Geometry: final body of the model. Coordinates: model frame, mm. A direction names the side the tool comes from. Give positions to 0.01 mm unless a question says otherwise; leave off trailing zeros. Write each loop counter-clockwise with the first axis right and the second up, starting at its lowest first coordinate (ties: lowest second). Pieces come first, ordered by that corner, then holes. Notation, with made-up numbers: M 12.25,66 L 22.25,66 A30 ccw 22.25,104 Z; hole C -22,65 d5. An arc over 180 degrees is marked long. Use a Markdown table: item, result. Add a question column.
(1) Cut plane D-D (x = 8). Output: boundary loops of the cut face in (y, z), plus the area to 3 significant figures.
(2) Material intervals for L1, parallel to Z at x = 9, y = 19.75; L2, parallel to Z at x = 18, y = 22.75; L3, parallel to X at y = 23.25, z = -15.5, sorted ascending.
(3) Draft query along Y for faces 6 (the flat face through (41.5, 2.5, -2)), 7 (the flat face through (22, 25, -14)), 8 (the flat face through (22, 23, -14)). Return one class per face: released by +Y, released by -Y, zero draft, split by the parting line, or undercut.
(4) Cut plane C-C (y = 14.75). Output: boundary loops of the cut face in (x, z), plus the area to 3 significant figures.
(5) Cut plane A-A (z = -11.5). Output: boundary loops of the cut face in (x, y).
(6) Reachability of faces 1 (the flat face through (44, 3, -14)), 2 (the flat face through (22.7, 22.5, -25)), 3 (the flat face through (41, 24, -26)), 4 (the flat face through (1, 7.21, -14)), 5 (the flat face through (22, 12, 0)) from +Z, -Z, +X, -X, +Y, -Y: full face, straight path, thin tool, end or side. Return the list, or none.
(7) Pin query (flat end, axial travel): pin 1 Ø4 at (y, z) = (18, -23.5) entering from +X; pin 2 Ø0.9 at (x, z) = (41.5, -10.5) entering from +Y. Return the tip coordinate at first contact, or that it passes through.
(8) Cut plane B-B (z = -23). Output: boundary loops of the cut face in (x, y), plus the area to 3 significant figures.
```python
from build123d import *

# Parameters (mm, degrees)
SKETCH1_W           = 45
SKETCH1_H           = 28
BOSS_EXTRUDE1_DEPTH = 3
BOSS_EXTRUDE2_DEPTH = 22
SKETCH4_W           = 45
SKETCH4_H           = 28
SKETCH4_W_2         = 3
SKETCH4_H_2         = 24
BOSS_EXTRUDE4_DEPTH = 2
SKETCH5_W           = 8.5
SKETCH5_H           = 3.5
CUT_EXTRUDE1_DEPTH  = 2
BOSS_EXTRUDE6_DEPTH = 1
SKETCH8_W           = 3
SKETCH8_H           = 24
CUT_EXTRUDE2_DEPTH  = 1


with BuildPart() as part:
    # Sketch1 → Boss-Extrude1 (new body)
    with BuildSketch(Plane(origin=(0, 0, 0), x_dir=(1, 0, 0), z_dir=(0, 1, 0))):
        with Locations((22.5, 14)):
            Rectangle(SKETCH1_W, SKETCH1_H)
    extrude(amount=BOSS_EXTRUDE1_DEPTH)

    # Sketch2 → Boss-Extrude2 (add)
    with BuildSketch(Plane(origin=(0, 3, 0), x_dir=(1, 0, 0), z_dir=(0, 1, 0))):
        Polygon((40, 26), (40, 28), (0, 28), (0, 0), (40, 0), (40, 2), (2, 2), (2, 26), align=None)
    extrude(amount=BOSS_EXTRUDE2_DEPTH)

    # Sketch4 → Boss-Extrude4 (add)
    with BuildSketch(Plane(origin=(0, 25, 0), x_dir=(1, 0, 0), z_dir=(0, 1, 0))):
        with Locations((22.5, 14)):
            Rectangle(SKETCH4_W, SKETCH4_H)
        with Locations((41.5, 14)):
            Rectangle(SKETCH4_W_2, SKETCH4_H_2, mode=Mode.SUBTRACT)
    extrude(amount=-BOSS_EXTRUDE4_DEPTH)

    # Sketch5 → Cut-Extrude1 (cut)
    with BuildSketch(Plane.ZY):
        with BuildLine():
            Line((-18.47, 5.25), (-18.47, 5.96))
            ThreePointArc((-18.47, 5.96), (-18.103883476, 6.843883476), (-17.22, 7.21))
            Line((-17.22, 7.21), (-10.78, 7.21))
            ThreePointArc((-10.78, 7.21), (-9.896116524, 6.843883476), (-9.53, 5.96))
            Line((-9.53, 5.96), (-9.53, 5.25))
            ThreePointArc((-9.53, 5.25), (-9.896116524, 4.366116524), (-10.78, 4))
            Line((-10.78, 4), (-17.22, 4))
            ThreePointArc((-17.22, 4), (-18.103883476, 4.366116524), (-18.47, 5.25))
        make_face()
        with Locations((-14, 10.25)):
            Rectangle(SKETCH5_W, SKETCH5_H)
    extrude(amount=-CUT_EXTRUDE1_DEPTH, mode=Mode.SUBTRACT)

    # Sketch7 → Boss-Extrude6 (add)
    with BuildSketch(Plane.XZ.offset(-23)):
        Polygon((40, -25), (5, -25), (5, -3), (40, -3), (40, -2), (2, -2), (2, -26), (40, -26), align=None)
    extrude(amount=BOSS_EXTRUDE6_DEPTH)

    # Sketch8 → Cut-Extrude2 (cut)
    with BuildSketch(Plane(origin=(0, 3, 0), x_dir=(1, 0, 0), z_dir=(0, 1, 0))):
        with Locations((41.5, 14)):
            Rectangle(SKETCH8_W, SKETCH8_H)
    extrude(amount=-CUT_EXTRUDE2_DEPTH, mode=Mode.SUBTRACT)


solid = part.part
```
Answer list:
| question | item | result |
|---|---|---|
| 1 | outline | M 0,-28 L 25,-28 L 25,0 L 0,0 Z; hole M 3,-26 L 22,-26 L 22,-25 L 23,-25 L 23,-3 L 22,-3 L 22,-2 L 3,-2 Z |
| 1 | area | 222 mm² |
| 2 | L1 | -28 to -26, -2 to 0 |
| 2 | L2 | -28 to -25, -3 to 0 |
| 2 | L3 | 0 to 40, 43 to 45 |
| 3 | face 6 | zero draft |
| 3 | face 7 | released by +Y |
| 3 | face 8 | undercut |
| 4 | outline | M 0,-28 L 40,-28 L 40,-26 L 2,-26 L 2,-2 L 40,-2 L 40,0 L 0,0 Z |
| 4 | area | 208 mm² |
| 5 | outline | M 0,0 L 45,0 L 45,3 L 43,3 L 43,2 L 40,2 L 40,3 L 2,3 L 2,4 L 0,4 Z; M 0,7.21 L 2,7.21 L 2,8.5 L 0,8.5 Z; M 0,12 L 2,12 L 2,22 L 5,22 L 5,23 L 40,23 L 40,25 L 0,25 Z; M 43,23 L 45,23 L 45,25 L 43,25 Z |
| 6 | face 1 | +Z, -Z, +X |
| 6 | face 2 | +X |
| 6 | face 3 | +Y |
| 6 | face 4 | +X, -X |
| 6 | face 5 | +Z, +X, -X, +Y, -Y |
| 7 | pin 1 | x = 2 |
| 7 | pin 2 | y = 2 |
| 8 | outline | M 0,0 L 45,0 L 45,3 L 43,3 L 43,2 L 40,2 L 40,3 L 2,3 L 2,22 L 5,22 L 5,23 L 40,23 L 40,25 L 0,25 Z; M 43,23 L 45,23 L 45,25 L 43,25 Z |
| 8 | area | 259 mm² |
